CAD build for the part. Positions are in the model's coordinates, mm. Round coordinates to 2 decimals unless told otherwise and drop trailing zeros. Loops run counter-clockwise (first coordinate to the right, second up) from the corner with the lowest first, then second, coordinate; pieces in that order, holes last.
Autodesk Inventor part; units mm, degrees
ref_plane "YZ Plane" through (0, 0, 0) normal (1, 0, 0) x (0, 1, 0)
ref_plane "XZ Plane" through (0, 0, 0) normal (0, 1, 0) x (-1, 0, 0)
ref_plane "XY Plane" through (0, 0, 0) normal (0, 0, 1) x (1, 0, 0)
sketch "スケッチ1" plane through (0, 0, 0) normal (0, 0, 1) x (1, 0, 0)
  circle A0 centre (0, 0) radius 4
  dimension "d13" = 8
extrude "押し出し1" add sketch "スケッチ1" along normal blind 13
sketch "スケッチ2" plane through (0, 0, 13) normal (0, 0, 1) x (1, 0, 0)
  point P0 (0, 0)
  point P1 (0, 0)
hole "穴1" at (0, 0, 13) direction (0, 0, -1) diameter 3.242 end through all
chamfer "面取り1" distance 0.2 angle 45 4 edges at (0, 1.621, 13) (0, 1.621, 0) (-4, 0, 13) (-4, 0, 0)
properties part number "unir-spacer1" material "鋼、炭素鋼"
Item 1: Cut at A-A (y = 0). List the corners of the cut face in (x, z), plus the area to 3 significant figures.
Verdict:
outline: (-4, 0.2) - (-3.8, 0) - (-1.82, 0) - (-1.62, 0.2) - (-1.62, 12.8) - (-1.82, 13) - (-3.8, 13) - (-4, 12.8) - close; (1.62, 0.2) - (1.82, 0) - (3.8, 0) - (4, 0.2) - (4, 12.8) - (3.8, 13) - (1.82, 13) - (1.62, 12.8) - close
area: 61.7 mm2
Item 2: Flat gauge pins, fed straight in: P1, Ø1, axis at y = -2.5, z = 11.5, coming from the +X side; P2, Ø2.5, axis at x = 0, y = 0, coming from the -Z side. Where does each tip first touch, or does it go through?
Verdict:
P1: stops at x = 3.46
P2: passes through
Item 3: Mould opens along X. For faces 1 (the cylindrical face through (-0.867, 3.905, 6.412)), 2 (the flat face through (2, 1, 0)), 3 (the cylindrical face through (1.438, -0.748, 6.412)) say: released by +X, released by -X, zero draft, split by the parting line, or undercut.
Verdict:
face 1: split by the parting line
face 2: zero draft
face 3: undercut
Item 4: Cut at C-C (z = 1.25). List the corners of the cut face in (x, y).
Verdict:
outline: circle Ø8 at (0, 0); hole circle Ø3.24 at (0, 0)
Item 5: Wall check: L1, parallel to Y at x = 0, z = 5.5; L2, parallel to X at y = 0.5, z = 9; L3, parallel to X at y = 1, z = 5.5. Give the ranges that are in metal, low to high.
Verdict:
L1: y = -4 to -1.62, 1.62 to 4
L2: x = -3.97 to -1.54, 1.54 to 3.97
L3: x = -3.87 to -1.28, 1.28 to 3.87
